Check sheet for the drawn part. Datum: minimum x, y, z corner. Units: mm. Coordinates: 2 decimals unless noted, no trailing zeros. Order: outer loops, then holes, each group sorted by start corner. A loop starts at its lowest first (then second) coordinate and runs counter-clockwise, first axis right, second up.
1. Cross-section at D-D (x = 22). Enter the section's corners in (y, z), then the cut area to 3 significant figures.
2. Draft check along X on the marked faces 1, 2 and 3. Enter one of: released by +X, released by -X, zero draft, split by the parting line, or undercut.
3. Gauge pin test, flat ends, axial feed: pin 1 Ø8 at (y, z) = (18.5, 80) entering from +X; pin 2 Ø1.8 at (x, y) = (24.5, 13) entering from -Z; pin 3 Ø2 at (x, z) = (22, 37) entering from +Y. Record the tip position at first contact, or that the pin passes through.
4. Cross-section at A-A (x = 13). Enter the section's corners in (y, z).
5. Thickness scan on line 1 (Y direction, x = 13, z = 1.6); line 2 (Y direction, x = 13, z = 27); line 3 (Z direction, x = 12.75, y = 24). Record the ranges inside material, lowest first.
6. Cross-section at C-C (z = 87). Enter the section's corners in (x, y).
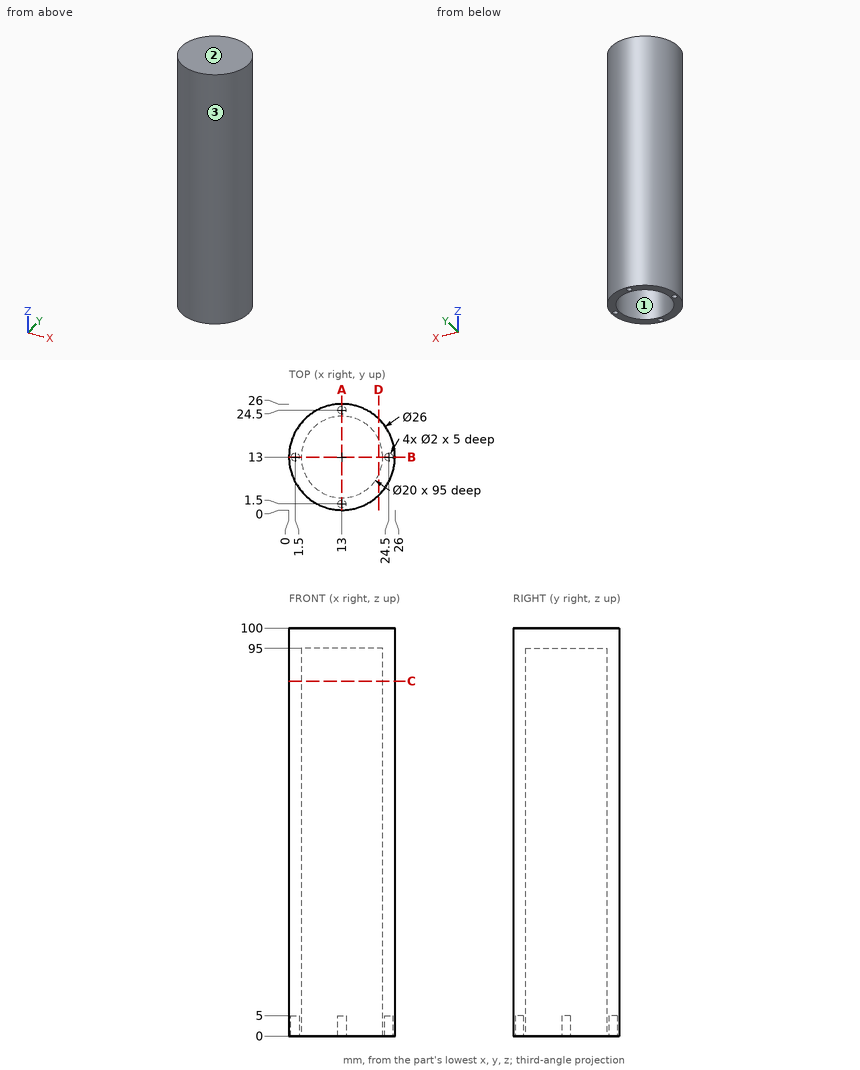
Data:
1. outline: (3.62, 0) - (8.64, 0) - (8.64, 95) - (17.36, 95) - (17.36, 0) - (22.38, 0) - (22.38, 100) - (3.62, 100) - close
1. area: 1,050 mm2
2. face 1: undercut
2. face 2: zero draft
2. face 3: split by the parting line
3. pin 1: stops at x = 25.91
3. pin 2: stops at z = 5
3. pin 3: stops at y = 23.25
4. outline: (0, 0) - (0.5, 0) - (0.5, 5) - (2.5, 5) - (2.5, 0) - (3, 0) - (3, 95) - (23, 95) - (23, 0) - (23.5, 0) - (23.5, 5) - (25.5, 5) - (25.5, 0) - (26, 0) - (26, 100) - (0, 100) - close
5. line 1: y = 0 to 0.5, 2.5 to 3, 23 to 23.5, 25.5 to 26
5. line 2: y = 0 to 3, 23 to 26
5. line 3: z = 5 to 100
6. outline: circle Ø26 at (13, 13); hole circle Ø20 at (13, 13)
